```python
from build123d import *

# Parameters (mm, degrees)
F0_W     = 118.554965
F0_H     = 87.894202
F1_DEPTH = 63.5
F2_W     = 105.414637
F2_H     = 76.505914
F3_DEPTH = 63.5
F5_DEPTH = 127
F6_R     = 10.184042
F7_DEPTH = 254


with BuildPart() as f1:
    # F0 (on Top) → F1 (new body)
    with BuildSketch(Plane.XY):
        with Locations((0.438012, -2.044052)):
            Rectangle(F0_W, F0_H)
    extrude(amount=F1_DEPTH)

    # F2 (on face) → F3 (cut)
    with BuildSketch(Plane.XY.offset(63.5)):
        with Locations((0.87602, -2.774071)):
            Rectangle(F2_W, F2_H)
    extrude(amount=-F3_DEPTH, mode=Mode.SUBTRACT)

    # F4 (on face) → F5 (cut)
    with BuildSketch(Plane.XZ.offset(45.991153)):
        Polygon((22.338558, 63.5), (-21.462537, 63.5), (-21.462537, 52.415308), (0.438012, 52.415308), (22.338558, 52.415308), align=None)
    extrude(amount=-F5_DEPTH, mode=Mode.SUBTRACT)

    # F6 (on face) → F7 (cut)
    with BuildSketch(Plane.YZ.offset(59.715495)):
        with Locations((0, 31.75)):
            Circle(F6_R)
    extrude(amount=-F7_DEPTH, mode=Mode.SUBTRACT)


solid = f1.part
```
The model under review builds one solid part; all positions refer to its coordinate system, in mm. A direction names the side the tool comes from. Round coordinates to 2 decimals unless told otherwise and drop trailing zeros. Write each loop counter-clockwise with the first axis right and the second up, starting at its lowest first coordinate (ties: lowest second). Pieces come first, ordered by that corner, then holes. Notation, with made-up numbers: (48.25, -13) - (54.25, -13) arc R18 cw to (54.25, 13) - close; hole circle Ø2 at (49, -7.75). An arc over 180 degrees is marked (long way). Answer as CSV lines item,"result". Start each with the question number.
(1) We need section A-A on y = -25. State the section outline as (x, z) points, plus the area to 3 significant figures.
(2) Draft analysis for pull direction Y (two halves, no side actions). For faces 4 (the flat face through (0, 41.903, 31)), 5 (the flat face through (0, 35.479, 32)), 6 (the flat face through (-51.831, -12, 32)), 7 (the flat face through (-53, 5, 63.5)), state which applies: pulls with the +Y half, pulls with the -Y half, needs draft (parallel to the pull), parting line crosses it, or undercut.
(3) We need section B-B on x = -9.5. State the section outline as (y, z) points, plus the area to 3 significant figures.
(4) For faces 1 (the flat face through (-21.463, -44, 58)), 2 (the flat face through (53.583, -12, 32)), 3 (the cylindrical face through (56.692, -1.326, 41.847)), list the 3-axis set-ups (+Z, -Z, +X, -X, +Y, -Y) from which the entire face can be reached by the end or side of a thin tool; tool diameter is ignored.
(5) For pin 1 Ø7 at (x, y) = (-9.5, 40) entering from +Z; pin 2 Ø10 at (x, y) = (-42.5, 10) entering from +Z, all flat-tipped, find the tip position at first contact; note any pin that passes through.
(6) We need section C-C on z = 54. State the section outline as (x, y) points, plus the area to 3 significant figures.
(7) To check wall thickness, follow line 1 (Y direction, x = 9, z = 44); line 2 (X direction, y = -15.5, z = 10.5); line 3 (Y direction, x = 55, z = 31). State the ranges of each line that lie inside material, in increasing order.
(8) We need section D-D on y = 0. State the section outline as (x, z) points.
Worked answers:
1,outline,"(-58.84, 0) - (-51.83, 0) - (-51.83, 63.5) - (-58.84, 63.5) - close; (53.58, 0) - (59.72, 0) - (59.72, 63.5) - (53.58, 63.5) - close"
1,area,"834 mm²"
2,face 4,"pulls with the +Y half"
2,face 5,"undercut"
2,face 6,"undercut"
2,face 7,"needs draft"
3,outline,"(-45.99, 0) - (-41.03, 0) - (-41.03, 52.42) - (-45.99, 52.42) - close; (35.48, 0) - (41.9, 0) - (41.9, 52.42) - (35.48, 52.42) - close"
3,area,"597 mm²"
4,face 1,"+Z, +Y, -Y"
4,face 2,"+Z, -Z"
4,face 3,"+X, -X"
5,pin 1,"z = 52.42"
5,pin 2,"through"
6,outline,"(-58.84, -45.99) - (-21.46, -45.99) - (-21.46, -41.03) - (-51.83, -41.03) - (-51.83, 35.48) - (-21.46, 35.48) - (-21.46, 41.9) - (-58.84, 41.9) - close; (22.34, -45.99) - (59.72, -45.99) - (59.72, 41.9) - (22.34, 41.9) - (22.34, 35.48) - (53.58, 35.48) - (53.58, -41.03) - (22.34, -41.03) - close"
6,area,"1,860 mm²"
7,line 1,"-45.99 to -41.03, 35.48 to 41.9"
7,line 2,"-58.84 to -51.83, 53.58 to 59.72"
7,line 3,"-45.99 to -10.16, 10.16 to 41.9"
8,outline,"(-58.84, 0) - (-51.83, 0) - (-51.83, 21.57) - (-58.84, 21.57) - close; (-58.84, 41.93) - (-51.83, 41.93) - (-51.83, 63.5) - (-58.84, 63.5) - close; (53.58, 0) - (59.72, 0) - (59.72, 21.57) - (53.58, 21.57) - close; (53.58, 41.93) - (59.72, 41.93) - (59.72, 63.5) - (53.58, 63.5) - close"
